Verification items for this drawing (mm, ordinates from the low corner). A direction names the side the tool comes from. Give positions to 0.01 mm unless a question says otherwise; leave off trailing zeros. Write each loop counter-clockwise with the first axis right and the second up, starting at its lowest first coordinate (ties: lowest second). Pieces come first, ordered by that corner, then holes. Notation, with made-up numbers: (7.5, -29) -> (42.5, -29) arc R18 cw to (42.5, -16) -> close; hole circle Ø7 at (53.5, -21). An arc over 180 degrees is marked (long way). One line per item, written item: value.
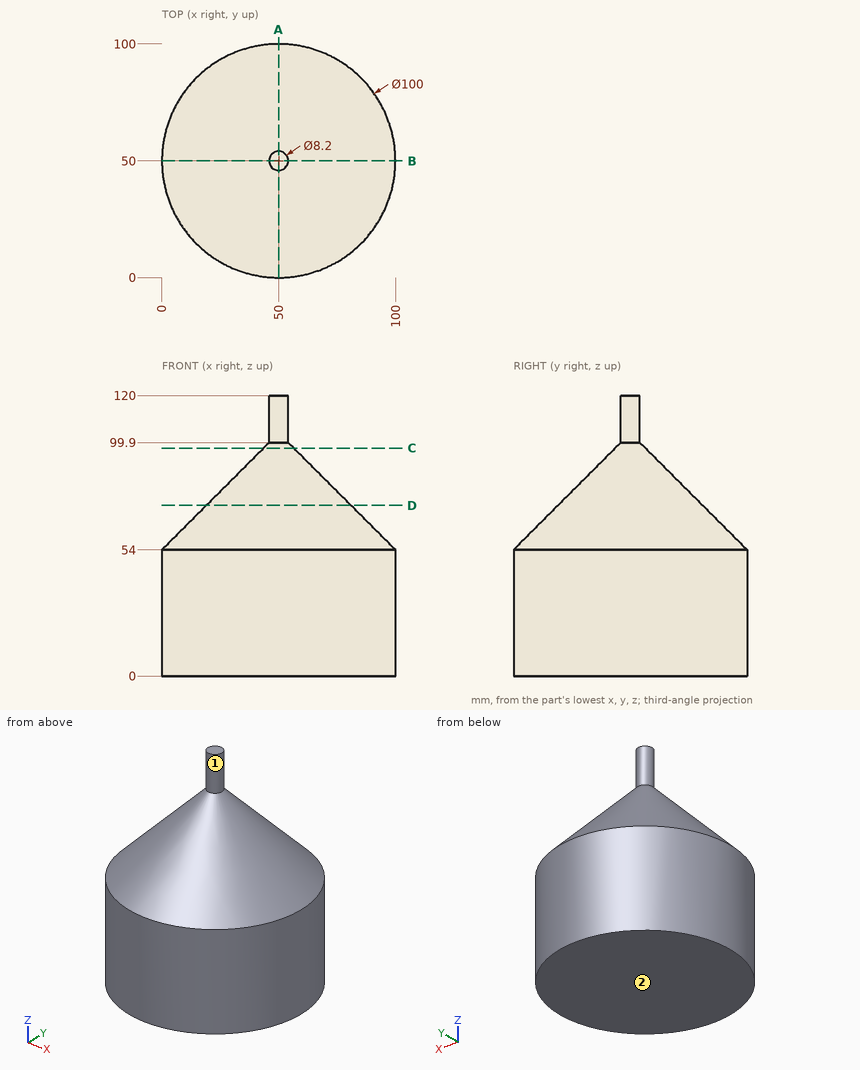
1) Tool access check on the marked faces 1 and 2. Record the directions out of +Z, -Z, +X, -X, +Y, -Y that give a thin tool (end or side, any length) a straight path to the whole face; none if there is none.
Verdict:
face 1: +Z
face 2: -Z, +X, -X, +Y, -Y
2) Sectioned sample at C-C on z = 97.5. Record the cut outline in (x, y).
Verdict:
outline: circle Ø13 at (50, 50)
3) Scan lines: probe 1 along Z at (x, y) = (36.5, 14); probe 2 along Y at (x, z) = (39, 58); probe 3 along Z at (x, y) = (31, 28). Record each from-to range of solid material in increasing order.
Verdict:
probe 1: 0 to 65.55
probe 2: 5.33 to 94.67
probe 3: 0 to 74.93
4) Sectioned sample at A-A on x = 50. Record the cut outline in (y, z), plus the area to 3 significant figures.
Verdict:
outline: (0, 0) -> (100, 0) -> (100, 54) -> (54.1, 99.9) -> (54.1, 120) -> (45.9, 120) -> (45.9, 99.9) -> (0, 54) -> close
area: 8,050 mm^2
5) Depth check by flat-ended pin: pin 1 Ø5 at (x, z) = (34, 46.5) entering from +Y; pin 2 Ø4 at (y, z) = (77, 57.5) entering from +X; pin 3 Ø5 at (x, z) = (42.5, 93) entering from +Y. Enter the tip coordinate at first touch or a pass-through.
Verdict:
pin 1: y = 98.14
pin 2: x = 90.63
pin 3: y = 61.6
6) Sectioned sample at D-D on z = 73. Record the cut outline in (x, y), plus the area to 3 significant figures.
Verdict:
outline: circle Ø62 at (50, 50)
area: 3,020 mm^2
